Answer from the drawing. Dimensions are ordinates in mm from the lowest x, y and z of the part. A direction names the side the tool comes from. Give positions to 0.01 mm unless a question says otherwise; leave off trailing zeros. Loops run counter-clockwise (first coordinate to the right, second up) from the corner with the lowest first, then second, coordinate; pieces in that order, holes last.
(1) Find section C-C, the plane z = 9.25. Write down the section's boundary in (x, y).
(2) Find section B-B, the plane x = 6.5. Write down the section's boundary in (y, z), then the cut area to 3 significant figures.
(3) Straight lines are drawn through the part: probe 1 along Z at (x, y) = (1, 8); probe 2 along Z at (x, y) = (1.75, 7); probe 3 along X at (y, z) = (3.25, 8). For each, find the intervals that lie inside material, in ascending order.
(4) Which of the six approach directions +Z, -Z, +X, -X, +Y, -Y give full straight-line access (tool end or side, diameter ignored) to the marked faces 1, 2 and 3?
(5) Find section D-D, the plane y = 3.25. Write down the section's boundary in (x, z), then the cut area to 3 significant figures.
(6) Find section A-A, the plane y = 5. Write down the section's boundary in (x, z).
(7) Each of these flat-tipped pins is pushed along its axis until it touches: P1, Ø1, axis at x = 7.5, z = 6, coming from the +Y side; P2, Ø6, axis at x = 6, y = 6, coming from the +Z side; P3, Ø2, axis at x = 9.5, y = 6.5, coming from the -Z side; P4, Ø4.5, axis at x = 11, y = 6, coming from the +Z side. Where does it stop, or does it pass through?
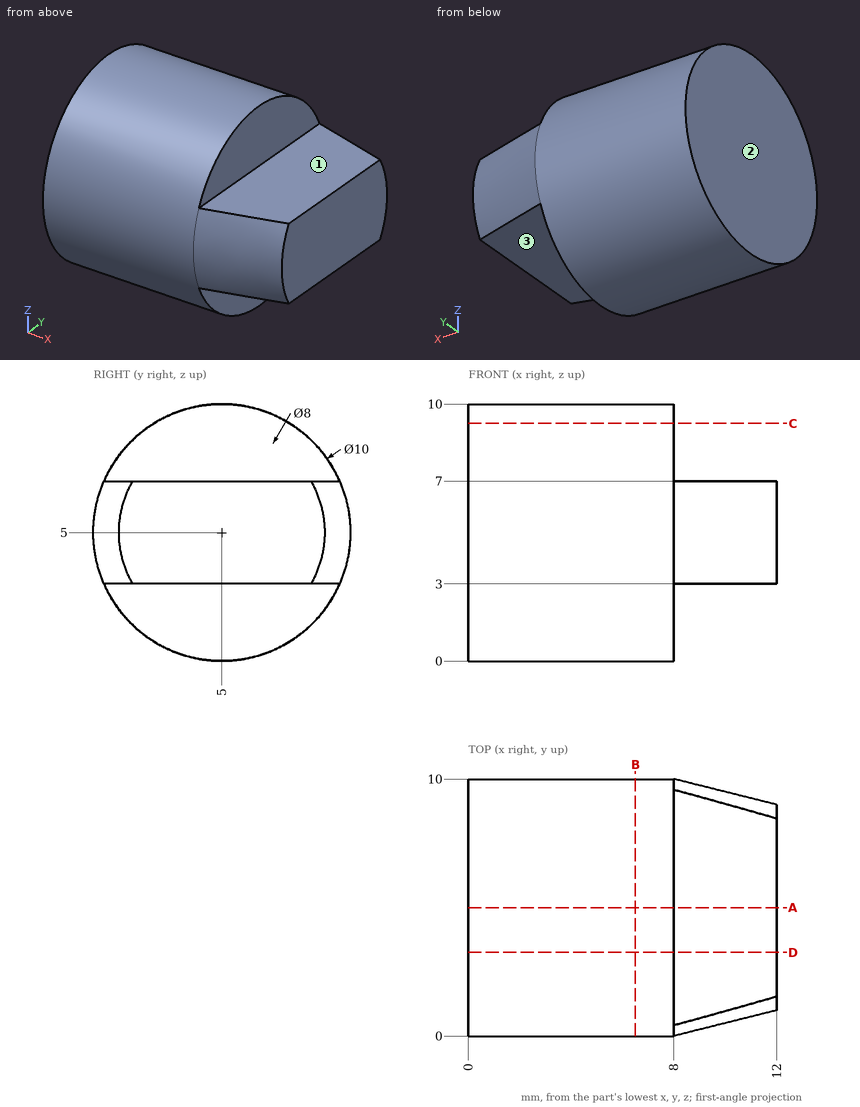
Entries:
1. outline: (0, 2.37) - (8, 2.37) - (8, 7.63) - (0, 7.63) - close
2. outline: circle Ø10 at (5, 5)
2. area: 78.5 mm2
3. probe 1: z = 1 to 9
3. probe 2: z = 0.42 to 9.58
3. probe 3: x = 0 to 8
4. face 1: +Z, +X, +Y, -Y
4. face 2: +Z, -Z, -X, +Y, -Y
4. face 3: -Z, +X, +Y, -Y
5. outline: (0, 0.32) - (8, 0.32) - (8, 3) - (12, 3) - (12, 7) - (8, 7) - (8, 9.68) - (0, 9.68) - close
5. area: 90.9 mm2
6. outline: (0, 0) - (8, 0) - (8, 3) - (12, 3) - (12, 7) - (8, 7) - (8, 10) - (0, 10) - close
7. P1: stops at y = 9.97
7. P2: stops at z = 10
7. P3: stops at z = 3
7. P4: stops at z = 7
